Geometry check sheet. Reference: the model listing, model coordinates, mm. Give positions to 0.01 mm unless a question says otherwise; leave off trailing zeros. Loops run counter-clockwise (first coordinate to the right, second up) from the corner with the lowest first, then second, coordinate; pieces in that order, holes last. Notation, with made-up numbers: (81, 35) - (98, 35) arc R28 cw to (98, 57) - close; hole circle Ø10 at (-11, 83.5). An arc over 180 degrees is marked (long way). Use a Markdown table: item, result. Add a question column.
1. Depth check by flat-ended pin: P1, Ø1.5, axis at y = 82, z = 2.5, coming from the -X side; P2, Ø0.6, axis at x = -3, z = 2, coming from the +Y side; P3, Ø1.5, axis at y = -81, z = 1, coming from the +X side. Enter the tip coordinate at first touch or a pass-through.
2. Cross-section at B-B on z = 1.4. Count the separate pieces of the cut face and the enclosed holes in it, and give its area (3 significant figures).
3. Cross-section at D-D on y = 63. Enter the section's corners in (x, z).
4. Material ranges on L1, parallel to Y at x = -2, z = 0.3; L2, parallel to Y at x = -29.5, z = 2.2; L3, parallel to Y at x = -88, z = 2 (3 decimals), recorded low to high.
5. Cross-section at A-A on x = -6.5. Enter the section's corners in (y, z).
6. Cross-section at C-C on x = -33. Enter the section's corners in (y, z), and give its area (3 significant figures).
from build123d import *

# Parameters (mm, degrees)
SKETCH3_W           = 180
SKETCH3_H           = 180
SKETCH3_W_2         = 20
SKETCH3_H_2         = 3.18
SKETCH3_W_3         = 19.75
BOSS_EXTRUDE1_DEPTH = 3.18
CUT_EXTRUDE1_DEPTH  = 128.318939675
SKETCH5_R           = 1.436023081
SKETCH5_W           = 3.18
SKETCH5_H           = 80.125
CUT_EXTRUDE2_DEPTH  = 128.318939675


with BuildPart() as part:
    # Sketch3 → Boss-Extrude1 (new body)
    with BuildSketch(Plane.XY):
        Rectangle(SKETCH3_W, SKETCH3_H)
        with Locations((-28.286899392, 36.024803222)):
            Rectangle(SKETCH3_W_2, SKETCH3_H_2, mode=Mode.SUBTRACT)
        with Locations((-0.125, -46.269729843)):
            Rectangle(SKETCH3_W_3, SKETCH3_H_2, mode=Mode.SUBTRACT)
    extrude(amount=BOSS_EXTRUDE1_DEPTH)

    # Sketch4 → Cut-Extrude1 (cut, through all)
    with BuildSketch(Plane.XY.offset(3.18)):
        Polygon((1.5, 86.82), (10, 86.82), (10, 90), (-10, 90), (-10, 86.82), (-1.5, 86.82), (-1.5, 82.82), (-3.5, 82.82), (-3.5, 79.82), (-1.5, 79.82), (-1.5, 77), (1.5, 77), (1.5, 79.82), (3.5, 79.82), (3.5, 82.82), (1.5, 82.82), align=None)
        Polygon((1.5, -79.82), (1.5, -77), (-1.5, -77), (-1.5, -79.82), (-3.5, -79.82), (-3.5, -82.82), (-1.5, -82.82), (-1.5, -86.82), (-10, -86.82), (-10, -90), (10, -90), (10, -86.82), (1.5, -86.82), (1.5, -82.82), (3.5, -82.82), (3.5, -79.82), align=None)
    extrude(amount=-CUT_EXTRUDE1_DEPTH, mode=Mode.SUBTRACT)

    # Sketch5 → Cut-Extrude2 (cut, through all)
    with BuildSketch(Plane.XY.offset(3.18)):
        with Locations((-88, 0)):
            Circle(SKETCH5_R)
        with Locations((88, 0)):
            Circle(SKETCH5_R)
        with Locations((-88.41, 49.9375)):
            Rectangle(SKETCH5_W, SKETCH5_H)
        with Locations((-88.41, -49.9375)):
            Rectangle(SKETCH5_W, SKETCH5_H)
        with Locations((88.41, -49.9375)):
            Rectangle(SKETCH5_W, SKETCH5_H)
        with Locations((88.41, 49.9375)):
            Rectangle(SKETCH5_W, SKETCH5_H)
    extrude(amount=-CUT_EXTRUDE2_DEPTH, mode=Mode.SUBTRACT)


solid = part.part
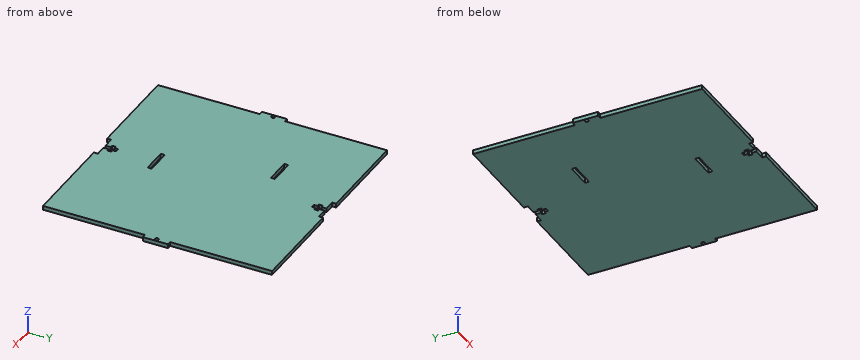
Values found:
| question | item | result |
|---|---|---|
| 1 | P1 | stops at x = -86.82 |
| 1 | P2 | stops at y = 86.82 |
| 1 | P3 | stops at x = 86.82 |
| 2 | separate pieces | 1 |
| 2 | enclosed holes | 4 |
| 2 | area | 31,000 mm2 |
| 3 | outline | (-86.82, 0) - (86.82, 0) - (86.82, 3.18) - (-86.82, 3.18) - close |
| 4 | L1 | y = -86.82 to -82.82, -79.82 to -47.86, -44.68 to 79.82, 82.82 to 86.82 |
| 4 | L2 | y = -90 to 34.43, 37.61 to 90 |
| 4 | L3 | y = -9.875 to -1.436, 1.436 to 9.875 |
| 5 | outline | (-86.82, 0) - (-47.86, 0) - (-47.86, 3.18) - (-86.82, 3.18) - close; (-44.68, 0) - (86.82, 0) - (86.82, 3.18) - (-44.68, 3.18) - close |
| 6 | outline | (-90, 0) - (34.43, 0) - (34.43, 3.18) - (-90, 3.18) - close; (37.61, 0) - (90, 0) - (90, 3.18) - (37.61, 3.18) - close |
| 6 | area | 562 mm2 |
